```python
from build123d import *

# Parameters (mm, degrees)
SALIENTE_EXTRUIR1_DEPTH = 8
SALIENTE_EXTRUIR2_DEPTH = 8
CROQUIS3_W              = 290
CROQUIS3_H              = 78
SALIENTE_EXTRUIR3_DEPTH = 2
SALIENTE_EXTRUIR4_REACH = 385.299
CROQUIS4_R              = 5
SALIENTE_EXTRUIR5_REACH = 385.299
CROQUIS5_R              = 5


with BuildPart() as part:
    # Croquis1 → Saliente-Extruir1 (new body)
    with BuildSketch(Plane.XY.offset(39)):
        with BuildLine():
            Line((-14.882678763, -17.53584537), (25.33811134, -51.671245521))
            ThreePointArc((25.33811134, -51.671245521), (34.318759969, -53.096192455), (39.715363545, -45.777777778))
            ThreePointArc((39.715363545, -45.777777778), (47.742688304, -29.553380316), (64.616402247, -23))
            Line((64.616402247, -23), (350, -23))
            ThreePointArc((350, -23), (373, 0), (350, 23))
            Line((350, 23), (0, 23))
            ThreePointArc((0, 23), (-21.590790207, 7.927028336), (-14.882678763, -17.53584537))
        make_face()
    extrude(amount=-SALIENTE_EXTRUIR1_DEPTH)



with BuildPart() as body_2:
    # Croquis2 → Saliente-Extruir2 (new body)
    with BuildSketch(Plane.XY.offset(-39)):
        with BuildLine():
            Line((-14.882678763, -17.53584537), (25.33811134, -51.671245521))
            ThreePointArc((25.33811134, -51.671245521), (34.318759969, -53.096192455), (39.715363545, -45.777777778))
            ThreePointArc((39.715363545, -45.777777778), (47.742688304, -29.553380316), (64.616402247, -23))
            Line((64.616402247, -23), (350, -23))
            ThreePointArc((350, -23), (373, 0), (350, 23))
            Line((350, 23), (0, 23))
            ThreePointArc((0, 23), (-21.590790207, 7.927028336), (-14.882678763, -17.53584537))
        make_face()
    extrude(amount=SALIENTE_EXTRUIR2_DEPTH)


with BuildPart() as part_1:
    add(part.part)

    add(body_2.part)  # Saliente-Extruir3 merges body 2
    # Croquis3 → Saliente-Extruir3 (add)
    with BuildSketch(Plane(origin=(0, 23, 0), x_dir=(1, 0, 0), z_dir=(0, 1, 0))):
        with Locations((189, 0)):
            Rectangle(CROQUIS3_W, CROQUIS3_H)
    extrude(amount=SALIENTE_EXTRUIR3_DEPTH)

    # Croquis4 → Saliente-Extruir4 (add, up to next)
    with BuildSketch(Plane.XY.offset(-31), mode=Mode.PRIVATE) as saliente_extruir4_sk1:
        Circle(CROQUIS4_R)
    saliente_extruir4_tool1 = extrude(saliente_extruir4_sk1.sketch, amount=SALIENTE_EXTRUIR4_REACH, mode=Mode.PRIVATE) - part_1.part
    add(saliente_extruir4_tool1.solids().sort_by_distance((0, 0, -31))[0])

    # Croquis5 → Saliente-Extruir5 (add, up to next)
    with BuildSketch(Plane(origin=(0, 0, 31), x_dir=(-1, 0, 0), z_dir=(0, 0, -1)), mode=Mode.PRIVATE) as saliente_extruir5_sk1:
        with Locations(Location((-350, 0, 0), (0, 0, 180))):
            Circle(CROQUIS5_R)
    saliente_extruir5_tool1 = extrude(saliente_extruir5_sk1.sketch, amount=SALIENTE_EXTRUIR5_REACH, mode=Mode.PRIVATE) - part_1.part
    add(saliente_extruir5_tool1.solids().sort_by_distance((350, 0, 31))[0])


solid = part_1.part
```
The model under review builds one solid part; all positions refer to its coordinate system, in mm. A direction names the side the tool comes from. Round coordinates to 2 decimals unless told otherwise and drop trailing zeros. Loops run counter-clockwise (first coordinate to the right, second up) from the corner with the lowest first, then second, coordinate; pieces in that order, holes last. Notation, with made-up numbers: M 83,17.5 L 91,17.5 A8 cw 91,27.5 Z; hole C 12.5,69.25 d11. An arc over 180 degrees is marked long. Put each result on its own line as item: value.
Q1. For pin 1 (1 mm diameter, centred on y = -6.5, z = -20.5, fed in from -X) (3 decimals); pin 2 (9 mm diameter, centred on x = 30.5, z = -33, fed in from +Y); pin 3 (6 mm diameter, centred on x = 151, z = 22, fed in from -Y); pin 4 (2.5 mm diameter, centred on x = 257.5, z = 34.5, fed in from -Y), all flat-tipped, find the tip position at first contact; note any pin that passes through.
Result set:
pin 1: passes through
pin 2: stops at y = 23
pin 3: stops at y = 23
pin 4: stops at y = -23
Q2. Consider section B-B, the plane z = 9. Give the boundary of the cut face in (x, y).
Result set:
outline: C 0,0 d10; M 44,23 L 334,23 L 334,25 L 44,25 Z; C 350,0 d10
Q3. Machinability: for faces 1 (the flat face through (22, 23, 35)), 2 (the flat face through (205, -23, -35)), 3 (the flat face through (187, 23, 0)), 4 (the flat face through (342, 23, 35)), which of the approach directions +Z, -Z, +X, -X, +Y, -Y give a long, thin tool a straight path to every point of the face, cutting with its end or side? Answer none if there is none.
Result set:
face 1: +Z, -Z, -X, +Y
face 2: +Z, -Z, +X, -Y
face 3: +X, -X, -Y
face 4: +Z, -Z, +X, +Y
Q4. Consider section A-A, the plane y = 0. Give the boundary of the cut face in (x, z), then the cut area to 3 significant figures.
Result set:
outline: M -23,-39 L 373,-39 L 373,-31 L 355,-31 L 355,31 L 373,31 L 373,39 L -23,39 L -23,31 L -5,31 L -5,-31 L -23,-31 Z; hole M 5,-31 L 345,-31 L 345,31 L 5,31 Z
area: 7,580 mm²
Q5. To check wall thickness, follow L1, parallel to Z at x = 26, y = -31.5; L2, parallel to X at y = -2, z = -19.5; L3, parallel to Y at x = 197, z = 16. State the ranges of each line that lie inside material, in increasing order.
Result set:
L1: z = -39 to -31, 31 to 39
L2: x = -4.58 to 4.58, 345.42 to 354.58
L3: y = 23 to 25
Q6. Mouldability with a two-part tool opening along Z and no side actions: class faces 5 (the cylindrical face through (-1.08, -4.88, -0.43)), 6 (the flat face through (172, 2, -31)), 7 (the flat face through (172, 3, 39)), 8 (the flat face through (205, -23, 35)) as released by +Z, released by -Z, zero draft, split by the parting line, or undercut.
Result set:
face 5: undercut
face 6: undercut
face 7: released by +Z
face 8: zero draft
Q7. Consider section C-C, the plane x = 158. Give the boundary of the cut face in (y, z), then the cut area to 3 significant figures.
Result set:
outline: M -23,-39 L 25,-39 L 25,39 L -23,39 L -23,31 L 23,31 L 23,-31 L -23,-31 Z
area: 892 mm²
Q8. Consider section D-D, the plane y = 16. Give the boundary of the cut face in (x, z).
Result set:
outline: M -16.52,-39 L 366.52,-39 L 366.52,-31 L -16.52,-31 Z; M -16.52,31 L 366.52,31 L 366.52,39 L -16.52,39 Z
